Input: part model. Units: mm. Frame: model coordinates. Face numbers are marked on the shaded views. A direction names the side the tool comes from. Round coordinates to 2 decimals unless told otherwise and drop trailing zeros. Loops run counter-clockwise (first coordinate to the right, second up) from the corner with the lowest first, then second, coordinate; pieces in that order, holes last.
1) Ray query, line 1 along X through (y, z) = (1, 38); line 2 along Y through (x, z) = (5.25, 113.5) (3 decimals); line 3 along Z through (x, y) = (12.7, 1.55) (3 decimals). Return the intervals inside material, ascending.
2) Section C-C, the plane x = 19.75. Return loops of the section in (y, z) (3 decimals), and give its area (3 significant figures).
3) Section B-B, the plane x = 12.7. Return loops of the section in (y, z) (1 decimal).
4) First-contact query: pin 1 (1.6 mm diameter, centred on x = 24.5, z = 69.5, fed in from -Y); pin 2 (8.5 mm diameter, centred on x = 12.7, z = 114.3, fed in from +Y) (3 decimals); pin 3 (8 mm diameter, centred on x = 18.5, y = 34.5, fed in from +Z) (3 decimals); pin 4 (10 mm diameter, centred on y = 14.5, z = 34.5, fed in from -X) (3 decimals). Flat tips, straight axial feed; report the tip coordinate or a pass-through.
5) Draft query along X for the marked faces 3, 4 and 5. Return one class per face: pulls with the +X half, pulls with the -X half, needs draft (parallel to the pull), parting line crosses it, or undercut.
6) Section A-A, the plane x = 5.5. Return loops of the section in (y, z) (3 decimals), and give its area (3 significant figures).
7) Access query for the marked faces 1 and 2. Directions: +Z, -Z, +X, -X, +Y, -Y. A direction counts if a zero-diameter tool reaches every point of the face in a straight line with its end or side. Return the directions, or none.
Autodesk Inventor part; units mm, degrees
ref_plane "YZ Plane" through (0, 0, 0) normal (1, 0, 0) x (0, 1, 0)
ref_plane "XZ Plane" through (0, 0, 0) normal (0, 1, 0) x (-1, 0, 0)
ref_plane "XY Plane" through (0, 0, 0) normal (0, 0, 1) x (1, 0, 0)
sketch "Sketch1" plane through (0, 0, 0) normal (0, 0, 1) x (1, 0, 0)
  line L0 (0, 0) -> (25.4, 0)
  line L1 (25.4, 0) -> (25.4, 50.8)
  line L2 (25.4, 50.8) -> (0, 50.8)
  line L3 (0, 50.8) -> (0, 0)
  line L4 (3.175, 3.175) -> (22.225, 3.175)
  line L5 (22.225, 3.175) -> (22.225, 47.625)
  line L6 (22.225, 47.625) -> (3.175, 47.625)
  line L7 (3.175, 47.625) -> (3.175, 3.175)
  dimension "d0" = 50.8
  dimension "d1" = 25.4
  dimension "d2" = 3.175
  dimension "d3" = 3.175
  dimension "d4" = 3.175
  dimension "d5" = 3.175
extrude "Extrusion1" add sketch "Sketch1" along normal blind 152.4
sketch "Sketch2" plane through (0, 0, 0) normal (0, -1, 0) x (1, 0, 0)
  line L0 (25.4, 152.4) -> (0, 152.4)
  line L1 (0, 0) -> (0, 152.4)
  line L2 (25.4, 0) -> (25.4, 152.4)
  line L3 (0, 152.4) -> (25.4, 127)
  circle A0 centre (12.7, 114.3) radius 3.175
  circle A1 centre (12.7, 38.1) radius 3.175
  dimension "d8" = 45
  dimension "d9" = 6.35
  dimension "d10" = 12.7
  dimension "d11" = 38.1
  dimension "d12" = 76.2
extrude "Extrusion2" cut sketch "Sketch2" against normal blind 3.175 contours A0 | A1
extrude "Extrusion3" cut sketch "Sketch2" against normal through all contours L2 L3 L0
sketch "Sketch3" plane through (0, 50.8, 0) normal (0, 1, 0) x (1, 0, 0)
  circle A0 centre (12.7, -114.3) radius 3.175
  circle A1 centre (12.7, -38.1) radius 3.175
  circle A2 centre (12.7, -38.1) radius 4.7625
  circle A3 centre (12.7, -114.3) radius 4.7625
  dimension "d17" = 9.525
extrude "Extrusion4" cut sketch "Sketch3" against normal blind 3.175 contours A0 | A1 | A2 | A3
sketch "Sketch4" plane through (25.4, 0, 0) normal (1, 0, 0) x (0, 0, -1)
  line L0 (-127, 50.8) -> (-127, 0)
  line L1 (0, 0) -> (-127, 0)
  line L2 (0, 0) -> (0, 50.8)
  line L3 (0, 50.8) -> (-127, 50.8)
  line L4 (0, 50.8) -> (0, 0)
  line L5 (-127, 50.8) -> (0, 50.8)
  line L6 (-127, 0) -> (-127, 50.8)
  line L7 (-127, 0) -> (0, 0)
  line L8 (-55.7727, 44.45) -> (-74.93, 12.5211)
  line L9 (-74.93, 6.35) -> (-52.07, 44.45) construction
  line L10 (-120.65, 6.35) -> (-6.35, 6.35)
  line L11 (-6.35, 44.45) -> (-120.65, 44.45)
  line L12 (-52.07, 38.2789) -> (-71.2273, 6.35)
  line L13 (-52.07, 44.45) -> (-29.21, 6.35) construction
  line L14 (-48.3673, 44.45) -> (-29.21, 12.5211)
  line L15 (-94.0873, 44.45) -> (-74.93, 12.5211)
  line L16 (-97.79, 44.45) -> (-74.93, 6.35) construction
  line L17 (-78.6327, 6.35) -> (-97.79, 38.2789)
  line L18 (-52.07, 38.2789) -> (-32.9127, 6.35)
  line L19 (-116.9473, 6.35) -> (-97.79, 38.2789)
  line L20 (-120.65, 44.45) -> (-120.65, 6.35)
  line L21 (-120.65, 6.35) -> (-97.79, 44.45) construction
  line L22 (-120.65, 12.5211) -> (-101.4927, 44.45)
  line L23 (-29.21, 12.5211) -> (-10.0527, 44.45)
  line L24 (-25.5073, 6.35) -> (-6.35, 38.2789)
  line L25 (-6.35, 6.35) -> (-6.35, 44.45)
  line L26 (-29.21, 6.35) -> (-6.35, 44.45) construction
  dimension "d20" = 30.964
  dimension "d21" = 61.928
  dimension "d22" = 61.928
  dimension "d23" = 61.928
  dimension "d24" = 61.928
  dimension "d25" = 3.175
  dimension "d26" = 3.175
  dimension "d27" = 3.175
  dimension "d28" = 3.175
  dimension "d29" = 3.175
  dimension "d30" = 3.175
  dimension "d31" = 3.175
  dimension "d32" = 3.175
  dimension "d33" = 3.175
  dimension "d34" = 3.175
  dimension "d35" = 6.35
  dimension "d36" = 6.35
  dimension "d37" = 6.35
  dimension "d38" = 6.35
extrude "Extrusion5" cut sketch "Sketch4" against normal blind 3.175 contours L8 L15 L11 | L11 L23 L14 | L22 L20 L11 | L25 L10 L24 | L19 L17 L10 | L10 L12 L18
sketch "Sketch5" plane through (0, 0, 0) normal (-1, 0, 0) x (0, 0, 1)
  line L0 (152.4, 0) -> (152.4, 50.8)
  line L1 (0, 50.8) -> (152.4, 50.8)
  line L2 (0, 50.8) -> (0, 0)
  line L3 (0, 0) -> (152.4, 0)
  line L4 (0, 0) -> (0, 50.8)
  line L5 (152.4, 0) -> (0, 0)
  line L6 (152.4, 50.8) -> (152.4, 0)
  line L7 (152.4, 50.8) -> (0, 50.8)
  line L8 (90.17, 39.0811) -> (66.1672, 6.35)
  line L9 (86.2328, 44.45) -> (62.23, 11.7189)
  line L10 (62.23, 6.35) -> (90.17, 44.45) construction
  line L11 (6.35, 6.35) -> (146.05, 6.35)
  line L12 (146.05, 44.45) -> (6.35, 44.45)
  line L13 (90.17, 44.45) -> (118.11, 6.35) construction
  line L14 (90.17, 39.0811) -> (114.1728, 6.35)
  line L15 (118.11, 11.7189) -> (142.1128, 44.45)
  line L16 (118.11, 6.35) -> (146.05, 44.45) construction
  line L17 (146.05, 6.35) -> (146.05, 44.45)
  line L18 (122.0472, 6.35) -> (146.05, 39.0811)
  line L19 (94.1072, 44.45) -> (118.11, 11.7189)
  line L20 (38.2272, 44.45) -> (62.23, 11.7189)
  line L21 (34.29, 44.45) -> (62.23, 6.35) construction
  line L22 (10.2872, 6.35) -> (34.29, 39.0811)
  line L23 (6.35, 44.45) -> (6.35, 6.35)
  line L24 (6.35, 6.35) -> (34.29, 44.45) construction
  line L25 (6.35, 11.7189) -> (30.3528, 44.45)
  line L26 (58.2928, 6.35) -> (34.29, 39.0811)
  dimension "d41" = 36.254
  dimension "d42" = 72.508
  dimension "d43" = 72.508
  dimension "d44" = 72.508
  dimension "d45" = 72.508
  dimension "d46" = 3.175
  dimension "d47" = 3.175
  dimension "d48" = 3.175
  dimension "d49" = 3.175
  dimension "d50" = 3.175
  dimension "d51" = 3.175
  dimension "d52" = 3.175
  dimension "d53" = 3.175
  dimension "d54" = 3.175
  dimension "d55" = 3.175
  dimension "d56" = 6.35
  dimension "d57" = 6.35
  dimension "d58" = 6.35
  dimension "d59" = 6.35
extrude "Extrusion6" cut sketch "Sketch5" against normal blind 3.175 contours L14 L11 L8 | L11 L22 L26 | L18 L17 L11 | L23 L12 L25 | L15 L19 L12 | L12 L9 L20
fillet "Fillet1" radius 3.175 36 edges at (1.5875, 11.7189, 6.35) (1.5875, 44.45, 6.35) (1.5875, 44.45, 30.3528) (1.5875, 39.0811, 34.29) (1.5875, 6.35, 10.2872) (1.5875, 6.35, 58.2928) (1.5875, 44.45, 38.2272) (1.5875, 11.7189, 62.23) (1.5875, 44.45, 86.2328) (1.5875, 39.0811, 90.17) (1.5875, 6.35, 66.1672) (1.5875, 6.35, 114.1728) (1.5875, 44.45, 94.1072) (1.5875, 44.45, 142.1128) (1.5875, 11.7189, 118.11) (1.5875, 39.0811, 146.05) (1.5875, 6.35, 122.0472) (1.5875, 6.35, 146.05) (23.8125, 44.45, 120.65) (23.8125, 44.45, 101.4927) (23.8125, 12.5211, 120.65) (23.8125, 6.35, 116.9473) (23.8125, 38.2789, 97.79) (23.8125, 6.35, 78.6327) (23.8125, 12.5211, 74.93) (23.8125, 44.45, 94.0873) (23.8125, 44.45, 55.7727) (23.8125, 38.2789, 52.07) (23.8125, 6.35, 71.2273) (23.8125, 6.35, 32.9127) (23.8125, 12.5211, 29.21) (23.8125, 44.45, 48.3673) (23.8125, 44.45, 10.0527) (23.8125, 38.2789, 6.35) (23.8125, 6.35, 25.5073) (23.8125, 6.35, 6.35)
equation "\"d3\" = d2"
equation "\"d4\" = d3"
equation "\"d5\" = d4"
equation "\"d21\" = 2 * d20"
equation "\"d22\" = d21"
equation "\"d23\" = d22"
equation "\"d24\" = d23"
equation "\"d26\" = d25"
equation "\"d27\" = d26"
equation "\"d28\" = d27"
equation "\"d29\" = d28"
equation "\"d30\" = d29"
equation "\"d31\" = d30"
equation "\"d32\" = d30"
equation "\"d33\" = d32"
equation "\"d34\" = d33"
equation "\"d42\" = 2 * d41"
equation "\"d43\" = d42"
equation "\"d44\" = d43"
equation "\"d45\" = d44"
equation "\"d47\" = d46"
equation "\"d48\" = d47"
equation "\"d49\" = d48"
equation "\"d50\" = d49"
equation "\"d51\" = d50"
equation "\"d52\" = d51"
equation "\"d53\" = d51"
equation "\"d54\" = d53"
equation "\"d55\" = d54"
properties part number "5in 1by2 frame"
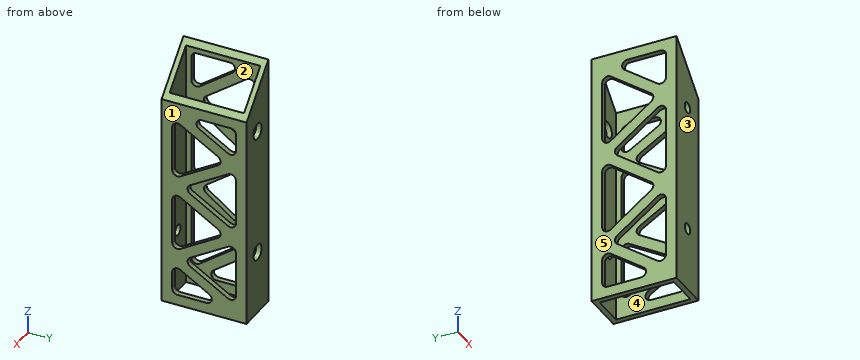
Final values:
1. line 1: x = 0 to 9.53, 15.87 to 25.4
1. line 2: y = 0 to 3.175, 47.625 to 50.8
1. line 3: z = 0 to 34.925, 41.275 to 111.125, 117.475 to 139.7
2. outline: (0, 0) - (3.175, 0) - (3.175, 132.65) - (0, 132.65) - close; (47.625, 0) - (50.8, 0) - (50.8, 132.65) - (47.625, 132.65) - close
2. area: 842 mm2
3. outline: (0, 0) - (3.2, 0) - (3.2, 34.9) - (0, 34.9) - close; (0, 41.3) - (3.2, 41.3) - (3.2, 111.1) - (0, 111.1) - close; (0, 117.5) - (3.2, 117.5) - (3.2, 139.7) - (0, 139.7) - close; (47.6, 0) - (50.8, 0) - (50.8, 33.3) - (47.6, 33.3) - close; (47.6, 42.9) - (50.8, 42.9) - (50.8, 109.5) - (47.6, 109.5) - close; (47.6, 119.1) - (50.8, 119.1) - (50.8, 139.7) - (47.6, 139.7) - close
4. pin 1: stops at y = 0
4. pin 2: stops at y = 3.175
4. pin 3: stops at z = 130.175
4. pin 4: stops at x = 22.225
5. face 3: needs draft
5. face 4: undercut
5. face 5: pulls with the -X half
6. outline: (0, 0) - (3.175, 0) - (3.175, 146.9) - (0, 146.9) - close; (47.625, 0) - (50.8, 0) - (50.8, 146.9) - (47.625, 146.9) - close
6. area: 933 mm2
7. face 1: +Z, -Z, +X, +Y, -Y
7. face 2: +Z, -Z
